Geometry check sheet. Reference: the model listing, model coordinates, mm. Face numbers are marked on the shaded views. A direction names the side the tool comes from. Coordinates: 2 decimals unless noted, no trailing zeros. Loops run counter-clockwise (first coordinate to the right, second up) from the corner with the lowest first, then second, coordinate; pieces in that order, holes last.
Autodesk Fusion 360 part; units mm, degrees
sketch "Skizze1" plane through (0, 0, 0) normal (0, 0, 1) x (1, 0, 0)
  line L0 (0, 0) -> (20.8, 0)
  line L1 (20.8, 0) -> (20.8, 72)
  line L2 (20.8, 72) -> (0, 72)
  line L3 (0, 72) -> (0, 0)
  dimension "d1" = 20.8
  dimension "d2" = 72
extrude "Extrusion1" add sketch "Skizze1" along normal blind 6
sketch "Skizze2" plane through (0, 0, 0) normal (-1, 0, 0) x (0, -1, 0)
  line L0 (-72, 0) -> (0, 0)
  line L1 (0, 0) -> (0, 6)
  line L2 (0, 6) -> (-72, 6)
  line L3 (-72, 6) -> (-72, 0)
  line L4 (-24.5, 0) -> (-12, 0)
  line L5 (-12, 0) -> (-12, 1)
  line L6 (-12, 1) -> (-10, 3)
  line L7 (-10, 3) -> (-10, 5)
  line L8 (-10, 5) -> (-26.5, 5)
  line L9 (-26.5, 5) -> (-26.5, 3)
  line L10 (-26.5, 3) -> (-24.5, 1)
  line L11 (-24.5, 1) -> (-24.5, 0)
  dimension "d5" = 16.5
  dimension "d6" = 1
  dimension "d7" = 1
  dimension "d8" = 45
  dimension "d9" = 45
  dimension "d10" = 2
  dimension "d11" = 2
  dimension "d12" = 2
  dimension "d13" = 10
extrude "Extrusion2" cut sketch "Skizze2" against normal through all contours L0 L4 L5 L6 L7 L8 L9 L10 L11
sketch "Skizze3" plane through (0, 0, 6) normal (0, 0, 1) x (-1, 0, 0)
  line L0 (0, -72) -> (0, 0)
  line L1 (0, 0) -> (-20.8, 0)
  line L2 (-20.8, 0) -> (-20.8, -72)
  line L3 (-20.8, -72) -> (0, -72)
  line L4 (0, -72) -> (-20.8, -72)
  line L5 (-20.8, -72) -> (-20.8, 0)
  line L6 (-20.8, 0) -> (0, 0)
  line L7 (0, 0) -> (0, -2)
  line L8 (0, -2) -> (-18.8, -2)
  line L9 (-18.8, -2) -> (-18.8, -70)
  line L10 (-18.8, -70) -> (0, -70)
  line L11 (0, -70) -> (0, -72)
  dimension "d15" = 2
  dimension "d16" = 2
  dimension "d17" = 2
extrude "Extrusion3" add sketch "Skizze3" along normal blind 8 contours L0 L1 L2 L3 L4 L5 L6 L7 L8 L9 L10 L11
sketch "Skizze4" plane through (0, 0, 14) normal (0, 0, 1) x (-1, 0, 0)
  line L0 (0, -70) -> (-18.8, -70)
  line L1 (-18.8, -70) -> (-18.8, -2)
  line L2 (-18.8, -2) -> (0, -2)
  line L3 (0, -70) -> (-18.8, -70)
  line L4 (-18.8, -70) -> (-18.8, -2)
  line L5 (-18.8, -2) -> (0, -2)
  line L6 (0, -2) -> (0, -1.2)
  line L7 (0, -1.2) -> (-19.6, -1.2)
  line L8 (-19.6, -1.2) -> (-19.6, -70.8)
  line L9 (-19.6, -70.8) -> (0, -70.8)
  line L10 (0, -70.8) -> (0, -70)
  dimension "d49" = 0.8
  dimension "d50" = 0.8
  dimension "d51" = 0.8
extrude "Extrusion4" add sketch "Skizze4" along normal blind 1
sketch "Skizze5" plane through (0, 0, 6) normal (0, 0, 1) x (-1, 0, 0)
  line L0 (0, -2) -> (-18.8, -2)
  line L1 (-18.8, -2) -> (-18.8, -70)
  line L2 (-18.8, -70) -> (0, -70)
  line L3 (0, -70) -> (0, -2)
  line L4 (-18.8, -70) -> (-10, -70)
  line L5 (-10, -70) -> (-10, -63.5)
  line L6 (-10, -63.5) -> (-18.8, -63.5)
  line L7 (-18.8, -63.5) -> (-18.8, -70)
  dimension "d25" = 10
  dimension "d26" = 6.5
extrude "Extrusion5" add sketch "Skizze5" along normal blind 9 contours L1 L2 L4 L5 L6 L7
sketch "Skizze7" plane through (0, 0, 0) normal (0, 0, -1) x (1, 0, 0)
  line L0 (20.8, -24.5) -> (0, -24.5)
  line L1 (0, -24.5) -> (0, -72)
  line L2 (0, -72) -> (20.8, -72)
  line L3 (20.8, -72) -> (20.8, -24.5)
  point P0 (14, -66.25)
  dimension "d31" = 14
  dimension "d32" = 5.75
hole "Bohrung1" at (14, 66.25, 0) direction (0, 0, 1) diameter 3.5 end through all counterbore diameter 6.5 counterbore depth 4
chamfer "Fase1" distance 1.5 angle 45 1 edges at (15.6316, 66.8828, 4)
sketch "Skizze8" plane through (0, 0, 6) normal (0, 0, 1) x (-1, 0, 0)
  line L0 (-18.8, -63.5) -> (-10, -63.5)
  line L1 (-10, -63.5) -> (-10, -70)
  line L2 (-10, -70) -> (0, -70)
  line L3 (0, -70) -> (0, -2)
  line L4 (0, -2) -> (-18.8, -2)
  line L5 (-18.8, -2) -> (-18.8, -63.5)
  line L6 (0, -2) -> (-5, -2)
  line L7 (-5, -2) -> (-5, -9.5)
  line L8 (-5, -9.5) -> (0, -9.5)
  line L9 (0, -9.5) -> (0, -2)
  dimension "d38" = 5
  dimension "d39" = 9.5
extrude "Extrusion6" add sketch "Skizze8" along normal blind 9 contours L3 L4 L6 L7 L8 L9
sketch "Skizze9" plane through (0, 0, 0) normal (0, 0, -1) x (1, 0, 0)
  line L0 (0, -12) -> (20.8, -12)
  line L1 (20.8, -12) -> (20.8, 0)
  line L2 (20.8, 0) -> (0, 0)
  line L3 (0, 0) -> (0, -12)
  point P0 (0, -4.5)
  dimension "d42" = 4.5
hole "Bohrung2" at (0, 4.5, 0) direction (0, 0, 1) diameter 3.5 depth 16 tip angle 180 counterbore diameter 6.5 counterbore depth 6
chamfer "Fase2" distance 1.5 angle 45 1 edges at (1.75, 4.5, 6)
fillet "Abrundung6" radius 2 1 edges at (18.8, 2, 10.5)
fillet "Abrundung2" radius 2.8 2 edges at (19.6, 1.2, 14.5) (19.6, 70.8, 14.5)
fillet "Abrundung4" radius 4 2 edges at (20.8, 0, 7) (20.8, 72, 7)
fillet "Abrundung5" radius 3 1 edges at (10, 63.5, 10.5)
mirror "Spiegeln1" about plane through (0, 0, 0) normal (1, 0, 0) of bodies 1 merged
sketch "Skizze11" plane through (0, 0, 6) normal (0, 0, 1) x (-1, 0, 0)
  line L0 (-18.8, -4) -> (-18.8, -63.5)
  line L1 (-18.8, -63.5) -> (-13, -63.5)
  arc A0 (-10, -66.5) -> (-13, -63.5) centre (-13, -66.5) ccw
  line L2 (-10, -66.5) -> (-10, -70)
  line L3 (-10, -70) -> (10, -70)
  line L4 (10, -70) -> (10, -66.5)
  arc A1 (13, -63.5) -> (10, -66.5) centre (13, -66.5) ccw
  line L5 (13, -63.5) -> (18.8, -63.5)
  line L6 (18.8, -63.5) -> (18.8, -4)
  line L7 (16.8, -2) -> (5, -2)
  line L8 (5, -2) -> (5, -9.5)
  line L9 (5, -9.5) -> (-5, -9.5)
  line L10 (-5, -9.5) -> (-5, -2)
  line L11 (-5, -2) -> (-16.8, -2)
  line L12 (-5, -2) -> (-18.8, -2)
  line L13 (-18.8, -2) -> (-18.8, -6)
  line L14 (-18.8, -6) -> (-5, -6)
  line L15 (-5, -6) -> (-5, -2)
  arc A2 (-16.8, -2) -> (-18.8, -4) centre (-16.8, -4) ccw
  arc A3 (18.8, -4) -> (16.8, -2) centre (16.8, -4) ccw
  dimension "d68" = 4
extrude "Extrusion7" add sketch "Skizze11" along normal blind 9 contours L0 L10 L11 L12 L13 L14 L15 A2 | L12 L13 A2
sketch "Skizze10" plane through (0, 0, 0) normal (0, -1, 0) x (1, 0, 0)
  line L0 (16.8, 0) -> (16.8, 14)
  line L1 (16.8, 14) -> (-16.8, 14)
  line L2 (-16.8, 14) -> (-16.8, 0)
  circle A0 centre (10, 14) radius 2.25
  line L3 (-16.8, 0) -> (16.8, 0)
  dimension "d66" = 4.5
  dimension "d67" = 10
extrude "Extrusion8" cut sketch "Skizze10" against normal blind 12 contours L1 A0 | L1 A0
chamfer "Fase5" distance 1 angle 45 3 edges at (7.9844, 3.6, 15) (12.0156, 3.6, 15) (7.9844, 3.6, 15)
sketch "Skizze16" plane through (20.8, 0, 0) normal (1, 0, 0) x (0, 1, 0)
  line L0 (68, 0) -> (68, 14)
  line L1 (68, 14) -> (4, 14)
  line L2 (4, 14) -> (4, 0)
  line L3 (4, 0) -> (12, 0)
  line L4 (12, 0) -> (12, 1)
  line L5 (12, 1) -> (10, 3)
  line L6 (10, 3) -> (10, 5)
  line L7 (10, 5) -> (26.5, 5)
  line L8 (26.5, 5) -> (26.5, 3)
  line L9 (26.5, 3) -> (24.5, 1)
  line L10 (24.5, 1) -> (24.5, 0)
  line L11 (24.5, 0) -> (68, 0)
  line L12 (5, 14) -> (31.5, 14)
  line L13 (31.5, 14) -> (31.5, 0)
  line L14 (31.5, 0) -> (5, 0)
  line L15 (5, 0) -> (5, 14)
  dimension "d100" = 5
  dimension "d101" = 5
extrude "Extrusion12" add sketch "Skizze16" along normal blind 4 contours L1 L3 L4 L5 L6 L7 L8 L9 L10 L11 L12 L13 L14 L15
sketch "Skizze17" plane through (0, 0, 14) normal (0, 0, 1) x (-1, 0, 0)
  line L0 (-12.25, -1.2) -> (-12.25, 0)
  line L1 (-12.25, 0) -> (-16.8, 0)
  arc A0 (-16.8, 0) -> (-20.8, -4) centre (-16.8, -4) ccw
  line L2 (-20.8, -4) -> (-20.8, -5)
  line L3 (-20.8, -5) -> (-24.8, -5)
  line L4 (-24.8, -5) -> (-24.8, -31.5)
  line L5 (-24.8, -31.5) -> (-20.8, -31.5)
  line L6 (-20.8, -31.5) -> (-20.8, -68)
  arc A1 (-20.8, -68) -> (-16.8, -72) centre (-16.8, -68) ccw
  line L7 (-16.8, -72) -> (16.8, -72)
  arc A2 (16.8, -72) -> (20.8, -68) centre (16.8, -68) ccw
  line L8 (20.8, -68) -> (20.8, -4)
  arc A3 (20.8, -4) -> (16.8, 0) centre (16.8, -4) ccw
  line L9 (16.8, 0) -> (-7.75, 0)
  line L10 (-7.75, 0) -> (-7.75, -1.2)
  line L11 (-7.75, -1.2) -> (16.8, -1.2)
  arc A4 (19.6, -4) -> (16.8, -1.2) centre (16.8, -4) ccw
  line L12 (19.6, -4) -> (19.6, -68)
  arc A5 (16.8, -70.8) -> (19.6, -68) centre (16.8, -68) ccw
  line L13 (16.8, -70.8) -> (-16.8, -70.8)
  arc A6 (-19.6, -68) -> (-16.8, -70.8) centre (-16.8, -68) ccw
  line L14 (-19.6, -68) -> (-19.6, -4)
  arc A7 (-18.8, -2.0404) -> (-19.6, -4) centre (-16.8, -4) ccw
  line L15 (-18.8, -2.0404) -> (-18.8, -2)
  line L16 (-18.8, -2) -> (-18.7596, -2)
  arc A8 (-16.8, -1.2) -> (-18.7596, -2) centre (-16.8, -4) ccw
  line L17 (-16.8, -1.2) -> (-12.25, -1.2)
  line L18 (-20.8, -29.25) -> (-23.8, -29.25)
  line L19 (-23.8, -29.25) -> (-23.8, -7.25)
  line L20 (-23.8, -7.25) -> (-20.8, -7.25)
  line L21 (-20.8, -7.25) -> (-20.8, -29.25)
  dimension "d104" = 1
  dimension "d105" = 22
  dimension "d106" = 2.25
  dimension "d107" = 2.25
  dimension "d108" = 3
extrude "Extrusion13" cut sketch "Skizze17" against normal blind 7 contours L18 L19 L20 L21
fillet "Abrundung11" radius 4 2 edges at (20.8, 5, 7) (20.8, 31.5, 7)
fillet "Abrundung12" radius 2 2 edges at (24.8, 5, 7) (24.8, 31.5, 7)
chamfer "Fase7" distance 1 angle 45 15 edges at (19.0361, 0.6834, 0) (21.6018, 4.0273, 0) (24.3723, 5.5944, 0) (24.8, 9.4152, 0) (-20.8, 8, 0) (-19.6284, 1.1716, 0) (0, 0, 0) (20.8, 51.75, 0) (19.6284, 70.8284, 0) (0, 72, 0) (-19.6284, 70.8284, 0) (-20.8, 46.25, 0) (24.8, 27.1716, 0) (24.433, 30.9978, 0) (21.534, 33.1906, 0)
equation "d1 = ( 41.6 / 2 ) * 1 mm"
equation "d106 = d107"
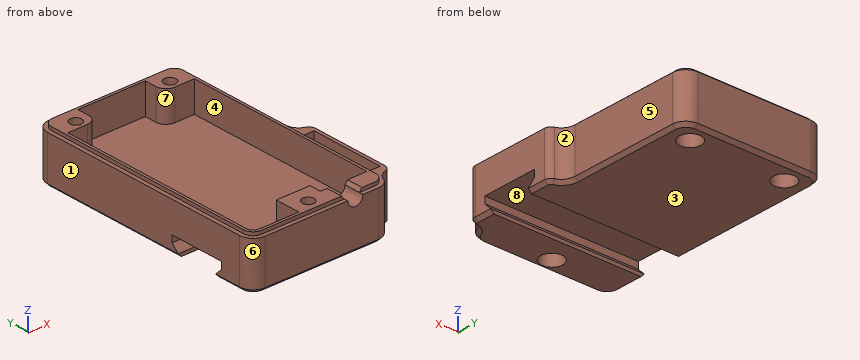
1) Access from +Z, -Z, +X, -X, +Y, -Y to the whole of each face (thin tool, end or side, straight path). Record for the marked faces 5, 6, 7 and 8.
Data:
face 5: +Z, -Z, +X, +Y
face 6: +Z, -Z, -X, -Y
face 7: +Z
face 8: +X, -X
2) Depth check by flat-ended pin: pin 1 (8 mm diameter, centred on x = 10.5, y = 18.5, fed in from -Z); pin 2 (6 mm diameter, centred on x = 14, y = 66.25, fed in from -Z); pin 3 (4 mm diameter, centred on y = 68, z = 12.5, fed in from +X); pin 4 (2 mm diameter, centred on x = 0, y = 4.5, fed in from -Z). Enter the tip coordinate at first touch or a pass-through.
Data:
pin 1: stops at z = 5
pin 2: stops at z = 4.25
pin 3: stops at x = 20.8
pin 4: passes through
3) Material ranges on probe 1 along X at (y, z) = (66.25, 8.5); probe 2 along X at (y, z) = (66.25, 2.25); probe 3 along Y at (x, z) = (0, 13), recorded low to high.
Data:
probe 1: x = -20.8 to -15.75, -12.25 to -10.01, 10.01 to 12.25, 15.75 to 20.8
probe 2: x = -20.8 to -17.25, -10.75 to 10.75, 17.25 to 20.8
probe 3: y = 0 to 2.75, 6.25 to 9.5, 70 to 72
4) Section check D-D on z = 8.5. Count the separate pieces of the cut face and the enclosed holes in it, and give its area (3 significant figures).
Data:
separate pieces: 1
enclosed holes: 5
area: 682 mm2
5) Section check B-B on y = 23.5. Record the cut outline in (x, z), and give its area (3 significant figures).
Data:
outline: (-20.8, 5) - (24.8, 5) - (24.8, 14) - (23.8, 14) - (23.8, 7) - (20.8, 7) - (20.8, 14) - (19.6, 14) - (19.6, 15) - (18.8, 15) - (18.8, 6) - (-18.8, 6) - (-18.8, 15) - (-19.6, 15) - (-19.6, 14) - (-20.8, 14) - close
area: 90.2 mm2
6) Mould release check, pull along X, two halves, no side actions. Record for the marked faces 1, 2, 3 and 4: +X half, -X half, draft (parallel to the pull), parting line (faces both ways), or undercut.
Data:
face 1: -X half
face 2: +X half
face 3: draft
face 4: undercut
